Verification items for the finished model (mm, model axes). Face numbers are marked on the shaded views. A direction names the side the tool comes from. Give positions to 0.01 mm unless a question says otherwise; leave off trailing zeros. Order: outer loops, then holes, each group sorted by start corner. A loop starts at its lowest first (then second) coordinate and runs counter-clockwise, first axis right, second up. Notation, with made-up numbers: (-28.5, 76) -> (12.5, 76) arc R12 ccw to (12.5, 98) -> close; hole circle Ø3 at (-26, 30.5). An arc over 180 degrees is marked (long way). One line per question, with ' | ' between items. Start each with the question number.
Q1. Section check C-C on y = 9.75. Record the cut outline in (x, z).
Q2. Material ranges on probe 1 along X at (y, z) = (-0.5, -4.75); probe 2 along X at (y, z) = (0.25, -1.5); probe 3 along Z at (x, y) = (18, 1.5), recorded low to high. Write a range as [from, to].
Q3. Section check D-D on x = 22.5. Record the cut outline in (y, z), plus the area to 3 significant figures.
Q4. Go/stop test with flat-tipped pins: pin 1 (5 mm diameter, centred on y = 9.5, z = -7.5, fed in from -X); pin 2 (5.5 mm diameter, centred on x = 3.5, y = 6, fed in from -Z); pin 3 (0.8 mm diameter, centred on y = -1, z = -2, fed in from +X). Record where each tip stops, or that it passes through.
Q5. Section check A-A on z = -7.5. Record the cut outline in (x, y).
Q6. Mould release check, pull along X, two halves, no side actions. Record for the marked faces 5, 6, 7 and 8: released by +X, released by -X, zero draft, split by the parting line, or undercut.
Q7. Access from +Z, -Z, +X, -X, +Y, -Y to the whole of each face (thin tool, end or side, straight path). Record for the marked faces 1, 2, 3 and 4.
Q8. Section check B-B on x = 4. Record the cut outline in (y, z), plus the area to 3 significant figures.
from build123d import *

# Parameters (mm, degrees)
SKETCH1_W                       = 26.5
SKETCH1_H                       = 6
BOSS_EXTRUDE1_DEPTH             = 17
SKETCH2_R                       = 1.5
CUT_EXTRUDE1_DEPTH              = 1
SKETCH3_R                       = 1.3
CUT_EXTRUDE2_DEPTH              = 32.878676259
SKETCH4_R                       = 3
CUT_EXTRUDE3_DEPTH              = 33.050741021
SKETCH5_R                       = 2.5
CUT_EXTRUDE4_DEPTH              = 1.5
SKETCH6_R                       = 1.5
CUT_EXTRUDE8_DEPTH              = 1
SKETCH7_R                       = 1.3
CUT_EXTRUDE9_DEPTH              = 32.678068123
CUT_EXTRUDE10_START             = -1
SKETCH8_R                       = 2.5
CUT_EXTRUDE10_DEPTH             = 1
CUT_EXTRUDE11_START             = -1
SKETCH9_R                       = 1.5
CUT_EXTRUDE11_DEPTH             = 1
SKETCH10_R                      = 5.5
SKETCH10_R_2                    = 3
BOSS_EXTRUDE2_DEPTH             = 3.5
SKETCH11_R                      = 3
SKETCH11_R_2                    = 1.3
BOSS_EXTRUDE4_DEPTH             = 2
CUT_EXTRUDE12_START             = -1
SKETCH12_R                      = 1.5
CUT_EXTRUDE12_DEPTH             = 1
SKETCH17_W                      = 2
SKETCH17_H                      = 6
BOSS_EXTRUDE6_DEPTH             = 1.5
SKETCH18_R                      = 1
CUT_EXTRUDE17_DEPTH             = 33.050741021
CHAMFER2_SIZE                   = 5
CHAMFER2_SIZE2                  = 3.5
FILLET11_R                      = 3
BOSS_EXTRUDE7_DEPTH             = 2
CUT_EXTRUDE19_DEPTH             = 33.050741021
FILLET13_R                      = 5
FILLET14_R                      = 3
FILLET15_R                      = 3
SKIZZE1_R                       = 0.5
SCHNITT_LINEAR_AUSTRAGEN1_DEPTH = 33.050741021


with BuildPart() as part:
    # Sketch1 → Boss-Extrude1 (new body)
    with BuildSketch(Plane(origin=(0, 0, 0), x_dir=(1, 0, 0), z_dir=(0, 1, 0))):
        with Locations((13.25, 3)):
            Rectangle(SKETCH1_W, SKETCH1_H)
    extrude(amount=BOSS_EXTRUDE1_DEPTH)

    # Sketch2 → Cut-Extrude1 (cut)
    with BuildSketch(Plane.XY):
        with Locations((12.5, 5.5)):
            Circle(SKETCH2_R)
    extrude(amount=-CUT_EXTRUDE1_DEPTH, mode=Mode.SUBTRACT)

    # Sketch3 → Cut-Extrude2 (cut, through all)
    with BuildSketch(Plane.XY.offset(-1)):
        with Locations((12.5, 5.5)):
            Circle(SKETCH3_R)
    extrude(amount=-CUT_EXTRUDE2_DEPTH, mode=Mode.SUBTRACT)

    # Sketch4 → Cut-Extrude3 (cut, through all)
    with BuildSketch(Plane.XY):
        with Locations((19.208203932, 11.5)):
            Circle(SKETCH4_R)
    extrude(amount=-CUT_EXTRUDE3_DEPTH, mode=Mode.SUBTRACT)

    # Sketch5 → Cut-Extrude4 (cut)
    with BuildSketch(Plane.XY):
        with Locations((3.5, 5.5)):
            Circle(SKETCH5_R)
    extrude(amount=-CUT_EXTRUDE4_DEPTH, mode=Mode.SUBTRACT)

    # Sketch6 → Cut-Extrude8 (cut)
    with BuildSketch(Plane.XY.offset(-1.5)):
        with Locations((3.5, 5.5)):
            Circle(SKETCH6_R)
    extrude(amount=-CUT_EXTRUDE8_DEPTH, mode=Mode.SUBTRACT)

    # Sketch7 → Cut-Extrude9 (cut, through all)
    with BuildSketch(Plane.XY.offset(-2.5)):
        with Locations((3.5, 5.5)):
            Circle(SKETCH7_R)
    extrude(amount=-CUT_EXTRUDE9_DEPTH, mode=Mode.SUBTRACT)

    # Sketch8 → Cut-Extrude10 (cut)
    with BuildSketch(Plane(origin=(0, 0, -6), x_dir=(-1, 0, 0), z_dir=(0, 0, -1)).offset(CUT_EXTRUDE10_START)):
        with Locations(Location((-3.5, 5.5, 0), (0, 0, 180))):
            Circle(SKETCH8_R)
    extrude(amount=CUT_EXTRUDE10_DEPTH, mode=Mode.SUBTRACT)

    # Sketch9 → Cut-Extrude11 (cut)
    with BuildSketch(Plane(origin=(0, 0, -5), x_dir=(-1, 0, 0), z_dir=(0, 0, -1)).offset(CUT_EXTRUDE11_START)):
        with Locations(Location((-3.5, 5.5, 0), (0, 0, 180))):
            Circle(SKETCH9_R)
    extrude(amount=CUT_EXTRUDE11_DEPTH, mode=Mode.SUBTRACT)

    # Sketch10 → Boss-Extrude2 (add)
    with BuildSketch(Plane(origin=(0, 0, -6), x_dir=(-1, 0, 0), z_dir=(0, 0, -1))):
        with Locations(Location((-19.208203932, 11.5, 0), (0, 0, 90))):
            Circle(SKETCH10_R)
        with Locations(Location((-19.208203932, 11.5, 0), (0, 0, 180))):
            Circle(SKETCH10_R_2, mode=Mode.SUBTRACT)
    extrude(amount=BOSS_EXTRUDE2_DEPTH)

    # Sketch11 → Boss-Extrude4 (add)
    with BuildSketch(Plane(origin=(0, 0, -6), x_dir=(-1, 0, 0), z_dir=(0, 0, -1))):
        with Locations(Location((-12.5, 5.5, 0), (0, 0, 180))):
            Circle(SKETCH11_R)
        with Locations(Location((-12.5, 5.5, 0), (0, 0, 180))):
            Circle(SKETCH11_R_2, mode=Mode.SUBTRACT)
    extrude(amount=BOSS_EXTRUDE4_DEPTH)

    # Sketch12 → Cut-Extrude12 (cut)
    with BuildSketch(Plane(origin=(0, 0, -8), x_dir=(-1, 0, 0), z_dir=(0, 0, -1)).offset(CUT_EXTRUDE12_START)):
        with Locations(Location((-12.5, 5.5, 0), (0, 0, 180))):
            Circle(SKETCH12_R)
    extrude(amount=CUT_EXTRUDE12_DEPTH, mode=Mode.SUBTRACT)

    # Sketch17 → Boss-Extrude6 (add)
    with BuildSketch(Plane.XZ):
        with Locations((6, -3)):
            Rectangle(SKETCH17_W, SKETCH17_H)
        with Locations((20.5, -3)):
            Rectangle(SKETCH17_W, SKETCH17_H)
    extrude(amount=BOSS_EXTRUDE6_DEPTH)

    # Sketch18 → Cut-Extrude17 (cut, through all)
    with BuildSketch(Plane(origin=(0, 0, -6), x_dir=(-1, 0, 0), z_dir=(0, 0, -1))):
        with Locations((-22.5, 0)):
            Circle(SKETCH18_R)
        with Locations((-18.5, 0)):
            Circle(SKETCH18_R)
        with Locations((-8, 0)):
            Circle(SKETCH18_R)
        with Locations((-4, 0)):
            Circle(SKETCH18_R)
    extrude(amount=-CUT_EXTRUDE17_DEPTH, mode=Mode.SUBTRACT)

    # Chamfer2
    chamfer2_edges = [part.edges().sort_by_distance(p)[0] for p in [
        (26.5, 17, -3),
    ]]
    chamfer2_side = [part.faces().sort_by_distance(p)[0] for p in [
        (26.5, 8.5, -3),
    ]]
    chamfer(chamfer2_edges, length=CHAMFER2_SIZE, length2=CHAMFER2_SIZE2, reference=chamfer2_side[0])

    # Fillet11
    fillet11_edges = [part.edges().sort_by_distance(p)[0] for p in [
        (23, 17, -3),
        (26.5, 12, -3),
    ]]
    fillet(fillet11_edges, radius=FILLET11_R)

    # Sketch19 → Boss-Extrude7 (add)
    with BuildSketch(Plane(origin=(0, 0, -6), x_dir=(-1, 0, 0), z_dir=(0, 0, -1))):
        with BuildLine():
            Line((-14.547099294, 14.419606745), (-9.957579288, 7.09251277))
            ThreePointArc((-9.957579288, 7.09251277), (-14.736067977, 7.5), (-13.800160725, 2.796376119))
            Line((-13.800160725, 2.796376119), (-21.591831928, 6.543356218))
            ThreePointArc((-21.591831928, 6.543356218), (-15.108745974, 7.833333333), (-14.547099294, 14.419606745))
        make_face()
    extrude(amount=BOSS_EXTRUDE7_DEPTH)

    # Sketch20 → Cut-Extrude19 (cut, through all)
    with BuildSketch(Plane(origin=(0, 0, -6), x_dir=(-1, 0, 0), z_dir=(0, 0, -1))):
        Polygon((0, 17), (-14.011012575, 17), (-9, 9), (0, 9), align=None)
    extrude(amount=-CUT_EXTRUDE19_DEPTH, mode=Mode.SUBTRACT)

    # Fillet13
    fillet13_edges = [part.edges().sort_by_distance(p)[0] for p in [
        (14.011012575, 17, -3),
    ]]
    fillet(fillet13_edges, radius=FILLET13_R)

    # Fillet14
    fillet14_edges = [part.edges().sort_by_distance(p)[0] for p in [
        (9, 9, -3),
    ]]
    fillet(fillet14_edges, radius=FILLET14_R)

    # Fillet15
    fillet15_edges = [part.edges().sort_by_distance(p)[0] for p in [
        (0, 9, -3),
    ]]
    fillet(fillet15_edges, radius=FILLET15_R)

    # Skizze1 → Schnitt-Linear austragen1 (cut, through all)
    with BuildSketch(Plane(origin=(0, 0, -6), x_dir=(-1, 0, 0), z_dir=(0, 0, -1))):
        with Locations((-23.5, 4)):
            Circle(SKIZZE1_R)
        with Locations((-7.5, 4)):
            Circle(SKIZZE1_R)
    extrude(amount=-SCHNITT_LINEAR_AUSTRAGEN1_DEPTH, mode=Mode.SUBTRACT)


solid = part.part
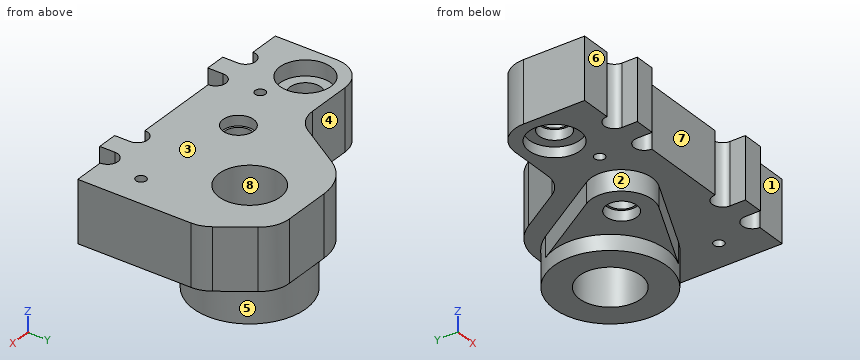
Filled in:
1) outline: (9.32, -6) -> (11.62, -6) -> (11.62, -8) -> (13.99, -8) -> (13.99, -9.5) -> (16.77, -9.5) -> (16.77, 0) -> (9.32, 0) -> close; (21.64, -9.5) -> (24.42, -9.5) -> (24.42, -6) -> (26.5, -6) -> (26.5, 0) -> (21.64, 0) -> close
2) probe 1: [5, 7], [19.5, 21.5] | probe 2: [0, 3.03], [4.97, 7.03], [8.97, 17.53], [19.47, 21.53], [23.47, 26.5] | probe 3: [-6, 0]
3) outline: (1, -6) -> (7.09, -6) -> (7.09, -9.5) -> (15.91, -9.5) -> (15.91, -6) -> (16.81, -6) -> (16.81, 0) -> (1, 0) -> close | area: 126 mm²
4) pin 1: x = 0.4 | pin 2: z = -6 | pin 3: x = 21.5
5) outline: (9.96, 7.09) arc R3 ccw to (13.8, 2.8) -> (21.59, 6.54) arc R5.5 ccw (long way) to (14.55, 14.42) -> close; hole circle Ø3 at (12.5, 5.5); hole circle Ø6 at (19.21, 11.5)
6) face 5: split by the parting line | face 6: zero draft | face 7: undercut | face 8: undercut
7) face 1: +Z, -Z, +X, -Y | face 2: -Z | face 3: +Z, +X, -X, +Y, -Y | face 4: +Z, -Z, -X, +Y
8) outline: (1, -6) -> (3.05, -6) -> (3.05, -5) -> (4.09, -5) -> (4.09, -4) -> (4.3, -4) -> (4.3, -2.5) -> (4.09, -2.5) -> (4.09, -1.5) -> (3.05, -1.5) -> (3.05, 0) -> (1, 0) -> close; (6.7, -4) -> (6.91, -4) -> (6.91, -5) -> (7.95, -5) -> (7.95, -6) -> (9, -6) -> (9, 0) -> (7.95, 0) -> (7.95, -1.5) -> (6.91, -1.5) -> (6.91, -2.5) -> (6.7, -2.5) -> close | area: 26.5 mm²
